Here's how the part is built. I have some questions about the finished solid (model axes, mm). A direction names the side the tool comes from. Round coordinates to 2 decimals unless told otherwise and drop trailing zeros. Loops run counter-clockwise (first coordinate to the right, second up) from the corner with the lowest first, then second, coordinate; pieces in that order, holes last. Notation, with made-up numbers: M 10,-15 L 58,-15 A17 ccw 58,3 Z; hole C -34,19 d9. An arc over 180 degrees is marked long. Use a Markdown table: item, result.
from build123d import *

# Parameters (mm, degrees)
CHAMFER1_SIZE      = 3.175
CHAMFER2_SIZE      = 1.5875
SKETCH2_R          = 3.175
CUT_EXTRUDE2_DEPTH = 72.490397082
CIRPATTERN2_COUNT  = 4
SKETCH3_R          = 2.38125
CUT_EXTRUDE3_DEPTH = 72.490397082


with BuildPart() as part:
    # Sketch1 → Revolve1 (revolve)
    with BuildSketch(Plane.XY, mode=Mode.PRIVATE) as revolve1_sk:
        Polygon((34.925, 0), (34.925, 3.175), (12.7, 3.175), (12.7, 12.7), (9.525, 12.7), (9.525, 41.275), (22.225, 41.275), (22.225, 9.525), (41.275, 9.525), (41.275, 0), align=None)
    revolve(revolve1_sk.sketch.rotate(Axis((0, 48.361075519, 0), (0, -1, 0)), 90), axis=Axis((0, 48.361075519, 0), (0, -1, 0)))

    # Chamfer1
    chamfer1_edges = [part.edges().sort_by_distance(p)[0] for p in [
        (0, 41.275, -9.525),
    ]]
    chamfer(chamfer1_edges, length=CHAMFER1_SIZE)

    # Chamfer2
    chamfer2_edges = [part.edges().sort_by_distance(p)[0] for p in [
        (0, 9.525, -41.275),
        (0, 9.525, -22.225),
        (0, 41.275, -22.225),
    ]]
    chamfer(chamfer2_edges, length=CHAMFER2_SIZE)

    # Sketch2 → Cut-Extrude2 (cut, through all)
    with BuildSketch(Plane(origin=(0, 41.275, 0), x_dir=(1, 0, 0), z_dir=(0, 1, 0))):
        with Locations(Location((28.575, 0, 0), (0, 0, 270))):
            Circle(SKETCH2_R)
    cut_extrude2 = extrude(amount=-CUT_EXTRUDE2_DEPTH, mode=Mode.SUBTRACT)

    # CirPattern2: Cut-Extrude2 ×4 about axis
    cirpattern2_axis = Axis((0, 0, 0), (0, 1, 0))
    for i in range(1, CIRPATTERN2_COUNT):
        add(cut_extrude2.rotate(cirpattern2_axis, i * 360 / CIRPATTERN2_COUNT), mode=Mode.SUBTRACT)

    # Sketch3 → Cut-Extrude3 (cut, through all)
    with BuildSketch(Plane(origin=(0, 0, 0), x_dir=(0, 0, -1), z_dir=(1, 0, 0))):
        with Locations(Location((0, 31.75, 0), (0, 0, 180))):
            Circle(SKETCH3_R)
    extrude(amount=CUT_EXTRUDE3_DEPTH, mode=Mode.SUBTRACT)


solid = part.part
1. For pin 1 Ø10 at (y, z) = (7.5, -20) entering from +X; pin 2 Ø7.5 at (x, z) = (0, -28.575) entering from +Y (3 decimals); pin 3 Ø8.5 at (x, z) = (0, 28.575) entering from -Y (3 decimals); pin 4 Ø5.5 at (x, z) = (28.575, 0) entering from -Y, each with a flat end and sliding along its axis, tell me the tip position at first contact or that it passes through.
Answer sheet:
| item | result |
|---|---|
| pin 1 | x = 38.45 |
| pin 2 | y = 9.525 |
| pin 3 | y = 3.175 |
| pin 4 | through |
2. We'd pull the mould along X, two halves only. Please class faces 6 (the face through (-40.924, 3.913, -5.373)), 7 (the face through (-9.444, 25.578, -1.24)), 8 (the face through (17, 9.525, -17)): +X half, -X half, draft (parallel to the pull), parting line (faces both ways), or undercut.
Answer sheet:
| item | result |
|---|---|
| face 6 | parting line |
| face 7 | undercut |
| face 8 | draft |
3. Which directions (+Z, -Z, +X, -X, +Y, -Y) give clear straight access to the entire face, cutting with the end or side of a thin tool? Please do faces 1 (the face through (-9, 0, -34)), 2 (the face through (15.63, 29.39, -0.31)), 3 (the face through (-15, 25.2, -16.4)), 4 (the face through (7.7, 8, -10.1)), 5 (the face through (25.476, 6.394, -0.688)).
Answer sheet:
| item | result |
|---|---|
| face 1 | +Z, -Z, +X, -X, -Y |
| face 2 | +X |
| face 3 | +Y |
| face 4 | -Y |
| face 5 | +Y, -Y |
4. Imagine slicing it at C-C, the plane y = 31.75. Write out the boundary of the cut face in (x, z) (3 decimals), then the cut area to 3 significant figures.
Answer sheet:
| item | result |
|---|---|
| outline | M 9.223,-2.381 A9.525 cw long 9.223,2.381 L 22.097,2.381 A22.225 ccw long 22.097,-2.381 Z |
| area | 1,210 mm2 |
5. Imagine slicing it at A-A, the plane x = 0. State how many separate pieces and enclosed holes the cut face has, then the cut area to 3 significant figures.
Answer sheet:
| item | result |
|---|---|
| separate pieces | 4 |
| enclosed holes | 0 |
| area | 1,100 mm2 |
6. I need wall thicknesses on probe 1 along X at (y, z) = (7, 0) (3 decimals); probe 2 along Y at (x, z) = (16.75, 0) (3 decimals); probe 3 along Y at (x, z) = (0, -19.5) (3 decimals). Which ranges of each line are inside material? Lowest first, please. Write a range as from..to.
Answer sheet:
| item | result |
|---|---|
| probe 1 | -41.275..-31.75, -25.4..-12.7, 12.7..25.4, 31.75..41.275 |
| probe 2 | 3.175..29.369, 34.131..41.275 |
| probe 3 | 3.175..41.275 |
